Verification items for this drawing (mm, ordinates from the low corner). A direction names the side the tool comes from. Coordinates: 2 decimals unless noted, no trailing zeros. Loops run counter-clockwise (first coordinate to the right, second up) from the corner with the lowest first, then second, coordinate; pieces in that order, holes last. Notation, with made-up numbers: (25, 31) -> (44, 31) arc R11 cw to (44, 49) -> close; hole circle Ø11 at (22, 44.25). An arc over 180 degrees is marked (long way). Write item = value, one per line.
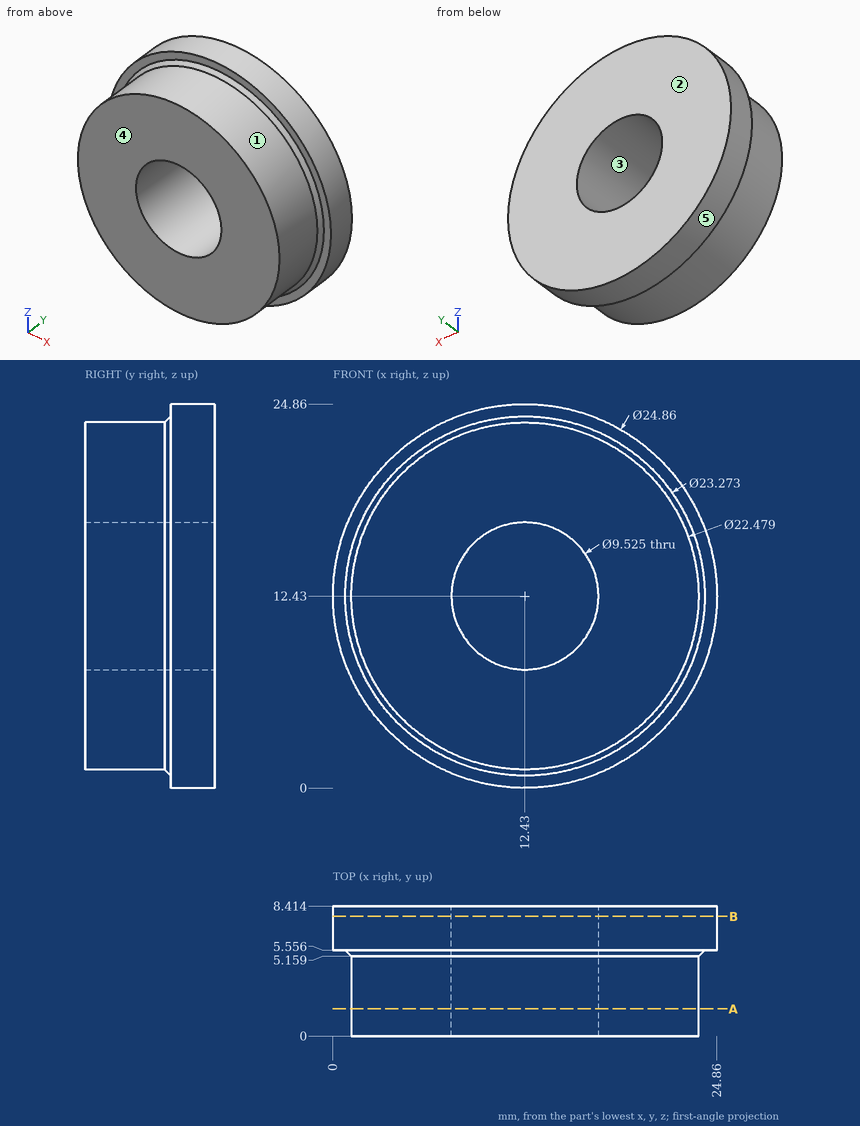
1) Tool access check on the marked faces 1 and 2. Record the directions out of +Z, -Z, +X, -X, +Y, -Y that give a thin tool (end or side, any length) a straight path to the whole face; none if there is none.
Ans:
face_1 = -Y
face_2 = +Z, -Z, +X, -X, +Y
2) Material ranges on line 1 (Y direction, x = 18, z = 23); line 2 (Z direction, x = 15.5, y = 1.5); line 3 (X direction, y = 5, z = 11.25) (1 decimal), recorded low to high.
Ans:
line_1 = 5.56 to 8.41
line_2 = 1.62 to 8.79, 16.07 to 23.24
line_3 = 1.3 to 7.8, 17 to 23.6
3) Depth check by flat-ended pin: pin 1 Ø1.5 at (y, z) = (4.5, 3) entering from -X; pin 2 Ø2 at (x, y) = (16.5, 2) entering from -Z; pin 3 Ø5 at (x, y) = (17.5, 2.5) entering from +Z. Enter the tip coordinate at first touch or a pass-through.
Ans:
pin_1 = 5.29
pin_2 = 1.62
pin_3 = 23.37
4) Sectioned sample at B-B, the plane y = 7.75. Record the cut outline in (x, z) (1 decimal), plus the area to 3 significant figures.
Ans:
outline = circle Ø24.9 at (12.4, 12.4); hole circle Ø9.5 at (12.4, 12.4)
area = 414 mm2
5) Sectioned sample at A-A, the plane y = 1.75. Record the cut outline in (x, z) (1 decimal), plus the area to 3 significant figures.
Ans:
outline = circle Ø22.5 at (12.4, 12.4); hole circle Ø9.5 at (12.4, 12.4)
area = 326 mm2
6) Release check for a two-part mould opening along Z. For the marked faces 3, 4 and 5 record: pulls with the +Z half, pulls with the -Z half, needs draft (parallel to the pull), parting line crosses it, or undercut.
Ans:
face_3 = undercut
face_4 = needs draft
face_5 = parting line crosses it
